Design review of the part built by this model. Coordinates are the model's own, in mm. A direction names the side the tool comes from. Coordinates: 2 decimals unless noted, no trailing zeros. Write each loop counter-clockwise with the first axis right and the second up, starting at its lowest first coordinate (ties: lowest second). Pieces come first, ordered by that corner, then holes.
Q1. Take a section at B-B (x = -4). Give the boundary of the cut face in (y, z), and give its area (3 significant figures).
Q2. Take a section at D-D (x = -9). Give the boundary of the cut face in (y, z).
Q3. Insertion check: pin 1 (1 mm diameter, centred on x = -7.5, y = 4, fed in from +Z); pin 2 (6 mm diameter, centred on x = 2.5, z = 38, fed in from +Y); pin 3 (2 mm diameter, centred on x = 0, y = -8.5, fed in from +Z); pin 4 (1.8 mm diameter, centred on x = 0, y = -8.3, fed in from -Z). Each pin has a flat end and moves straight along its axis. Give the tip position at first contact, or say it passes through.
Q4. Mouldability with a two-part tool opening along Y and no side actions: class faces 6 (the flat face through (5, -5, 0)), 7 (the cylindrical face through (-0.596, -2.685, 25.195)), 8 (the cylindrical face through (0.217, -7.324, 44.32)) as pulls with the +Y half, pulls with the -Y half, needs draft (parallel to the pull), parting line crosses it, or undercut.
Q5. Machinability: for faces 1 (the flat face through (-0.1, -3.3, 17.5)), 2 (the cylindrical face through (6.264, 3.767, -2.028)), 3 (the flat face through (0, 0, 35)), 4 (the flat face through (0, -7, 46.5)), 5 (the cylindrical face through (-2.38, -10.74, -2.03)), which of the approach directions +Z, -Z, +X, -X, +Y, -Y give a long, thin tool a straight path to every point of the face, cutting with its end or side? Answer none if there is none.
Q6. For probe 1 along Z at (x, y) = (3.5, 2.25); probe 2 along Y at (x, z) = (0, 43.7); probe 3 along Z at (x, y) = (-6.5, -1.5), list the stretches that pass through material, from the lowest coordinate up.
Q7. Take a section at C-C (y = -8.3). Give the boundary of the cut face in (x, z).
Q8. Take a section at A-A (y = 9.25). Give the boundary of the cut face in (x, z).
```python
from build123d import *

# Parameters (mm, degrees)
MOUNTING_FLANGE_START                          = -4
SKETCH1_R                                      = 11
MOUNTING_FLANGE_DEPTH                          = 4
SKETCH2_R                                      = 2.75
D5P5_CENTRAL_POST_DEPTH                        = 32.81
CLOSED_FLOOR_BELOW_SHAFT_NOSE_START            = 32.8
SKETCH3_R                                      = 10
CLOSED_FLOOR_BELOW_SHAFT_NOSE_DEPTH            = 2.2
SHAFT_AND_CLIP_CLEARANCE_START                 = 35
SKETCH4_R                                      = 10
SKETCH4_R_2                                    = 5.7
SHAFT_AND_CLIP_CLEARANCE_DEPTH                 = 6.5
LOWER_686ZZ_SEAT_START                         = 41.5
SKETCH5_R                                      = 10
SKETCH5_R_2                                    = 6.5
LOWER_686ZZ_SEAT_DEPTH                         = 5
SKETCH6_R                                      = 1
BASE_THREE_M2_THROUGH_THREAD_MAJOR_ENVEL_DEPTH = 4.01
TOP_CAP_THREE_M2_BLIND_THREAD_MAJOR_ENVE_START = -4.3
SKETCH7_R                                      = 1
TOP_CAP_THREE_M2_BLIND_THREAD_MAJOR_ENVE_DEPTH = 4.3
SKETCH8_R                                      = 6
BENCH_D12_ROOT_TO8P5_DEPTH                     = 8.5
BENCH_D10_MID_COLLAR_12P5_TO17P5_START         = 12.5
SKETCH9_R                                      = 5
BENCH_D10_MID_COLLAR_12P5_TO17P5_DEPTH         = 5
BENCH_STEP_TRANSITIONS_FILLET_R0P30_R          = 0.3


with BuildPart() as part:
    # Sketch1 → Mounting_Flange (new body)
    with BuildSketch(Plane.XY.offset(MOUNTING_FLANGE_START)):
        Circle(SKETCH1_R)
    extrude(amount=MOUNTING_FLANGE_DEPTH)

    # Sketch2 → D5p5_Central_Post (add)
    with BuildSketch(Plane.XY):
        Circle(SKETCH2_R)
    extrude(amount=D5P5_CENTRAL_POST_DEPTH)

    # Sketch3 → Closed_Floor_Below_Shaft_Nose (add)
    with BuildSketch(Plane.XY.offset(CLOSED_FLOOR_BELOW_SHAFT_NOSE_START)):
        Circle(SKETCH3_R)
    extrude(amount=CLOSED_FLOOR_BELOW_SHAFT_NOSE_DEPTH)

    # Sketch4 → Shaft_And_Clip_Clearance (add)
    with BuildSketch(Plane.XY.offset(SHAFT_AND_CLIP_CLEARANCE_START)):
        Circle(SKETCH4_R)
        with Locations(Location((0, 0, 0), (0, 0, 180))):
            Circle(SKETCH4_R_2, mode=Mode.SUBTRACT)
    extrude(amount=SHAFT_AND_CLIP_CLEARANCE_DEPTH)

    # Sketch5 → Lower_686ZZ_Seat (add)
    with BuildSketch(Plane.XY.offset(LOWER_686ZZ_SEAT_START)):
        Circle(SKETCH5_R)
        Circle(SKETCH5_R_2, mode=Mode.SUBTRACT)
    extrude(amount=LOWER_686ZZ_SEAT_DEPTH)

    # Sketch6 → Base_Three_M2_Through_Thread_Major_Envelopes (cut)
    with BuildSketch(Plane(origin=(0, 0, -4), x_dir=(-1, 0, 0), z_dir=(0, 0, -1))):
        with Locations((-7.188010851, 4.15)):
            Circle(SKETCH6_R)
        with Locations((7.188010851, 4.15)):
            Circle(SKETCH6_R)
        with Locations((0, -8.3)):
            Circle(SKETCH6_R)
    extrude(amount=-BASE_THREE_M2_THROUGH_THREAD_MAJOR_ENVEL_DEPTH, mode=Mode.SUBTRACT)

    # Sketch7 → Top_Cap_Three_M2_Blind_Thread_Major_Envelopes (cut)
    with BuildSketch(Plane.XY.offset(46.5).offset(TOP_CAP_THREE_M2_BLIND_THREAD_MAJOR_ENVE_START)):
        with Locations(Location((7.188010851, 4.15, 0), (0, 0, 180))):
            Circle(SKETCH7_R)
        with Locations(Location((-7.188010851, 4.15, 0), (0, 0, 180))):
            Circle(SKETCH7_R)
        with Locations(Location((0, -8.3, 0), (0, 0, 180))):
            Circle(SKETCH7_R)
    extrude(amount=TOP_CAP_THREE_M2_BLIND_THREAD_MAJOR_ENVE_DEPTH, mode=Mode.SUBTRACT)

    # Sketch8 → Bench_D12_Root_To8p5 (add)
    with BuildSketch(Plane.XY):
        Circle(SKETCH8_R)
    extrude(amount=BENCH_D12_ROOT_TO8P5_DEPTH)

    # Sketch9 → Bench_D10_Mid_Collar_12p5_To17p5 (add)
    with BuildSketch(Plane.XY.offset(BENCH_D10_MID_COLLAR_12P5_TO17P5_START)):
        Circle(SKETCH9_R)
    extrude(amount=BENCH_D10_MID_COLLAR_12P5_TO17P5_DEPTH)

    # Bench_Step_Transitions_Fillet_R0p30
    bench_step_transitions_fillet_r0p30_edges = [part.edges().sort_by_distance(p)[0] for p in [
        (-2.75, 0, 8.5),
        (-2.75, 0, 12.5),
        (-2.75, 0, 17.5),
    ]]
    fillet(bench_step_transitions_fillet_r0p30_edges, radius=BENCH_STEP_TRANSITIONS_FILLET_R0P30_R)


solid = part.part
```
Response:
1. outline: (-10.25, -4) - (10.25, -4) - (10.25, 0) - (4.47, 0) - (4.47, 8.5) - (-4.47, 8.5) - (-4.47, 0) - (-10.25, 0) - close; (-9.17, 32.8) - (9.17, 32.8) - (9.17, 46.5) - (5.12, 46.5) - (5.12, 41.5) - (4.06, 41.5) - (4.06, 35) - (-4.06, 35) - (-4.06, 41.5) - (-5.12, 41.5) - (-5.12, 46.5) - (-9.17, 46.5) - close; (-3, 12.5) - (3, 12.5) - (3, 17.5) - (-3, 17.5) - close
1. area: 335 mm2
2. outline: (-6.32, -4) - (6.32, -4) - (6.32, 0) - (-6.32, 0) - close; (-4.36, 32.8) - (4.36, 32.8) - (4.36, 46.5) - (-4.36, 46.5) - close
3. pin 1: stops at z = 42.2
3. pin 2: stops at y = 10
3. pin 3: stops at z = 46.5
3. pin 4: stops at z = 32.8
4. face 6: needs draft
4. face 7: parting line crosses it
4. face 8: undercut
5. face 1: none
5. face 2: -Z
5. face 3: +Z
5. face 4: +Z, +X, -X, +Y, -Y
5. face 5: +Z, -Z
6. probe 1: z = -4 to 8.5, 12.5 to 17.5, 32.8 to 35
6. probe 2: y = -10 to -9.3, -7.3 to -6.5, 6.5 to 10
6. probe 3: z = -4 to 0, 32.8 to 46.5
7. outline: (-7.22, -4) - (-1, -4) - (-1, 0) - (-7.22, 0) - close; (-5.58, 32.8) - (5.58, 32.8) - (5.58, 46.5) - (1, 46.5) - (1, 42.2) - (-1, 42.2) - (-1, 46.5) - (-5.58, 46.5) - close; (1, -4) - (7.22, -4) - (7.22, 0) - (1, 0) - close
8. outline: (-5.95, -4) - (5.95, -4) - (5.95, 0) - (-5.95, 0) - close; (-3.8, 32.8) - (3.8, 32.8) - (3.8, 46.5) - (-3.8, 46.5) - close
